Autodesk Inventor part; units mm, degrees
ref_plane "YZ Plane" through (0, 0, 0) normal (1, 0, 0) x (0, 1, 0)
ref_plane "XZ Plane" through (0, 0, 0) normal (0, 1, 0) x (-1, 0, 0)
ref_plane "XY Plane" through (0, 0, 0) normal (0, 0, 1) x (1, 0, 0)
sketch "Sketch1" plane through (0, 0, 0) normal (0, 1, 0) x (-1, 0, 0)
  arc A0 (-2.1541, 5.6) -> (2.1541, 5.6) centre (0, 0) ccw
  circle A1 centre (0, 0) radius 4.5
  line L0 (0, 5.6) -> (2.1541, 5.6)
  line L1 (0, 5.6) -> (-2.1541, 5.6)
  line L2 (0, 5.6) -> (3.5069, 5.6) construction
  line L3 (2.5, 2.9) -> (-2.5, 2.9)
  line L4 (-2.5, 2.9) -> (-2.5, 2.1)
  line L5 (-2.5, 2.1) -> (2.5, 2.1)
  line L6 (2.5, 2.1) -> (2.5, 2.9)
  line L7 (-2.5, -2.9) -> (2.5, -2.9)
  line L8 (2.5, -2.9) -> (2.5, -2.1)
  line L9 (2.5, -2.1) -> (-2.5, -2.1)
  line L10 (-2.5, -2.1) -> (-2.5, -2.9)
  line L11 (-2.5, 2.5) -> (2.5, 2.5)
  line L12 (-2.5, -2.5) -> (2.5, -2.5)
  line L13 (-4.5, 0) -> (4.5, 0)
  dimension "d0" = 12
  dimension "d1" = 9
  dimension "d2" = 180
  dimension "d3" = 4.3081
  dimension "d8" = 5
  dimension "d9" = 0.8
  dimension "d10" = 5
  dimension "d11" = 0.8
  dimension "d16" = 2.5
  dimension "d17" = 2.5
extrude "Extrusion1" add sketch "Sketch1" along normal blind 5.8 contours L1 L0 A0
extrude "Extrusion2" add sketch "Sketch1" along normal blind 12.8 contours L13 A1 | A1 L13 | L6 L11 L4 L3 | L6 L5 L4 L11 | L10 L12 L8 L7 | L10 L9 L8 L12
extrude "Extrusion3" add sketch "Sketch1" against normal blind 5 contours L6 L11 L4 L3 | L6 L5 L4 L11 | L10 L12 L8 L7 | L10 L9 L8 L12
properties part number "D6R90 F1 LFS"
Geometry: final body of the model. Coordinates: model frame, mm. A direction names the side the tool comes from. Coordinates: 2 decimals unless noted, no trailing zeros. Loops run counter-clockwise (first coordinate to the right, second up) from the corner with the lowest first, then second, coordinate; pieces in that order, holes last. Notation, with made-up numbers: M 76,-39.5 L 92,-39.5 A27 cw 92,-22.5 Z; hole C 40,63 d6. An arc over 180 degrees is marked long. One line per item, written item: value. Start each with the question number.
1) Material intervals for L1, parallel to Y at x = 1.5, z = 3.25; L2, parallel to Y at x = -4.25, z = 3.25; L3, parallel to X at y = 11.75, z = -3.5, sorted ascending. Write a range as from..to.
2) Cut plane C-C (z = 0). Return loops of the section in (x, y), then the cut area to 3 significant figures.
3) Pin query (flat end, axial travel): P1, Ø2.5, axis at x = 0, y = -3, coming from the -Z side; P2, Ø2.5, axis at x = 0.5, y = -3, coming from the +Z side; P3, Ø1.5, axis at x = 1, y = 3.5, coming from the -Z side; P4, Ø6, axis at x = -3, y = 0, coming from the +Z side. Return the tip coordinate at first contact, or that it passes through.
4) Cut plane B-B (x = 0). Return loops of the section in (y, z).
5) Cut plane A-A (y = -0.75). Return loops of the section in (x, z).
6) Cut plane D-D (y = 8.25). Return loops of the section in (x, z).
7) Reachability of faces 1 (the cylindrical face through (0, 3, -6)), 2 (the flat face through (0, -2, -2.1)), 3 (the cylindrical face through (0.59, 9.25, -4.46)), 4 (the flat face through (0, -2, -2.9)), 5 (the flat face through (0, -2, 2.9)) from +Z, -Z, +X, -X, +Y, -Y: full face, straight path, thin tool, end or side. Return the list, or none.
Evaluation:
1. L1: 0..12.8
1. L2: 0..5.8
1. L3: -2.83..2.83
2. outline: M -6,0 L 6,0 L 6,5.8 L 4.5,5.8 L 4.5,12.8 L -4.5,12.8 L -4.5,5.8 L -6,5.8 Z
2. area: 133 mm^2
3. P1: z = -2.9
3. P2: z = 2.9
3. P3: z = -5.99
3. P4: z = 5.6
4. outline: M -5,-2.9 L 0,-2.9 L 0,-6 L 5.8,-6 L 5.8,-4.5 L 12.8,-4.5 L 12.8,4.5 L 5.8,4.5 L 5.8,5.6 L 0,5.6 L 0,2.9 L -5,2.9 L -5,2.1 L 0,2.1 L 0,-2.1 L -5,-2.1 Z
5. outline: M -2.5,-2.9 L 2.5,-2.9 L 2.5,-2.1 L -2.5,-2.1 Z; M -2.5,2.1 L 2.5,2.1 L 2.5,2.9 L -2.5,2.9 Z
6. outline: C 0,0 d9
7. face 1: +Y, -Y
7. face 2: +X, -X, -Y
7. face 3: +Y
7. face 4: -Z, +X, -X, -Y
7. face 5: +Z, +X, -X, -Y
